```python
from build123d import *

# Parameters (mm, degrees)
SKETCH2_W           = 32.5
SKETCH2_H           = 32.5
SKETCH2_R           = 1
BOSS_EXTRUDE1_DEPTH = 1.5
SKETCH4_W           = 13
SKETCH4_H           = 13
BOSS_EXTRUDE2_DEPTH = 4
SKETCH6_W           = 10
SKETCH6_H           = 4.75
BOSS_EXTRUDE3_DEPTH = 6


with BuildPart() as part:
    # Sketch2 → Boss-Extrude1 (new body)
    with BuildSketch(Plane.XY):
        Rectangle(SKETCH2_W, SKETCH2_H)
        with Locations((13.875, 13.875)):
            Circle(SKETCH2_R, mode=Mode.SUBTRACT)
        with Locations((13.875, -13.875)):
            Circle(SKETCH2_R, mode=Mode.SUBTRACT)
        with Locations((-13.875, -13.875)):
            Circle(SKETCH2_R, mode=Mode.SUBTRACT)
        with Locations((-13.875, 13.875)):
            Circle(SKETCH2_R, mode=Mode.SUBTRACT)
    extrude(amount=BOSS_EXTRUDE1_DEPTH)

    # Sketch4 → Boss-Extrude2 (add)
    with BuildSketch(Plane.XY.offset(1.5)):
        Rectangle(SKETCH4_W, SKETCH4_H)
        with BuildLine():
            Line((8.925, -1.85), (-8.925, -1.85))
            ThreePointArc((-8.925, -1.85), (-10.775, 0), (-8.925, 1.85))
            Line((-8.925, 1.85), (8.925, 1.85))
            ThreePointArc((8.925, 1.85), (10.775, 0), (8.925, -1.85))
        make_face()
    extrude(amount=BOSS_EXTRUDE2_DEPTH)

    # Sketch5 → Revolve1 (revolve)
    with BuildSketch(Plane(origin=(0, 0, 0), x_dir=(1, 0, 0), z_dir=(0, 1, 0)), mode=Mode.PRIVATE) as revolve1_sk:
        with BuildLine():
            Line((0, -5.5), (6.5, -5.5))
            Line((6.5, -5.5), (6.5, -13.4))
            Line((6.5, -13.4), (5.65, -13.4))
            Line((5.65, -13.4), (5.65, -18.4))
            Line((5.65, -18.4), (8.5, -18.4))
            Line((8.5, -18.4), (8.5, -22.9))
            Line((8.5, -22.9), (7.5, -22.9))
            Line((7.5, -22.9), (7.5, -22.190584114))
            ThreePointArc((7.5, -22.190584114), (3.76673834, -22.722251095), (0, -22.9))
            Line((0, -22.9), (0, -5.5))
        make_face()
    revolve(revolve1_sk.sketch.rotate(Axis((0, 0, 0), (0, 0, 1)), 180), axis=Axis((0, 0, 0), (0, 0, 1)))

    # Sketch6 → Boss-Extrude3 (add)
    with BuildSketch(Plane(origin=(0, 0, 0), x_dir=(-1, 0, 0), z_dir=(0, 0, -1))):
        with Locations((0, -13.875)):
            Rectangle(SKETCH6_W, SKETCH6_H)
    extrude(amount=BOSS_EXTRUDE3_DEPTH)


solid = part.part
```
Geometry check sheet. Reference: the model listing, model coordinates, mm. A direction names the side the tool comes from. Coordinates: 2 decimals unless noted, no trailing zeros. Order: outer loops, then holes, each group sorted by start corner. A loop starts at its lowest first (then second) coordinate and runs counter-clockwise, first axis right, second up.
Item 1: Mould release check, pull along Y, two halves, no side actions. Record for faces 5 (the flat face through (0, 0, 0)), 6 (the flat face through (0, -11.5, -3)), 7 (the cylindrical face through (-4.032, -6.324, 22.54)): released by +Y, released by -Y, zero draft, split by the parting line, or undercut.
Item 2: Section check A-A (y = 0). Enter the section's corners in (x, z) (3 decimals).
Item 3: Section check C-C (z = 4.75). Enter the section's corners in (x, y) (3 decimals).
Item 4: Section check D-D (y = 3.5). Enter the section's corners in (x, z), plus the area to 3 significant figures.
Item 5: Tool access check on faces 1 (the flat face through (8, -1.85, 3)), 2 (the flat face through (-8, 1.85, 3)), 3 (the flat face through (2, 6, 18.4)), 4 (the flat face through (0, -6.5, 3)). Record the directions out of +Z, -Z, +X, -X, +Y, -Y that give a thin tool (end or side, any length) a straight path to the whole face; none if there is none.
Item 6: Depth check by flat-ended pin: pin 1 (1 mm diameter, centred on x = -2.5, z = -1, fed in from +Y); pin 2 (2.5 mm diameter, centred on x = -13.875, y = 13.875, fed in from +Z); pin 3 (1.9 mm diameter, centred on x = -8, z = 3.5, fed in from -Y). Enter the tip coordinate at first touch or a pass-through.
Item 7: Scan lines: line 1 along Y through (x, z) = (-14, 0.25); line 2 along Z through (x, y) = (1.5, -8); line 3 along Y through (x, z) = (-13, 1). Record each from-to range of solid material in increasing order.
Check sheet entries:
1. face 5: zero draft
1. face 6: released by +Y
1. face 7: undercut
2. outline: (-16.25, 0) - (16.25, 0) - (16.25, 1.5) - (10.775, 1.5) - (10.775, 5.5) - (6.5, 5.5) - (6.5, 13.4) - (5.65, 13.4) - (5.65, 18.4) - (8.5, 18.4) - (8.5, 22.9) - (7.5, 22.9) - (7.5, 22.191) arc R40 ccw to (-7.5, 22.191) - (-7.5, 22.9) - (-8.5, 22.9) - (-8.5, 18.4) - (-5.65, 18.4) - (-5.65, 13.4) - (-6.5, 13.4) - (-6.5, 5.5) - (-10.775, 5.5) - (-10.775, 1.5) - (-16.25, 1.5) - close
3. outline: (-8.925, -1.85) - (-6.5, -1.85) - (-6.5, -6.5) - (6.5, -6.5) - (6.5, -1.85) - (8.925, -1.85) arc R1.85 ccw to (8.925, 1.85) - (6.5, 1.85) - (6.5, 6.5) - (-6.5, 6.5) - (-6.5, 1.85) - (-8.925, 1.85) arc R1.85 ccw to start
4. outline: (-16.25, 0) - (16.25, 0) - (16.25, 1.5) - (6.5, 1.5) - (6.5, 5.5) - (5.48, 5.5) - (5.48, 13.4) - (4.44, 13.4) - (4.44, 18.4) - (7.75, 18.4) - (7.75, 22.9) - (6.63, 22.9) - (6.63, 22.19) arc R39.85 ccw to (-6.63, 22.19) - (-6.63, 22.9) - (-7.75, 22.9) - (-7.75, 18.4) - (-4.44, 18.4) - (-4.44, 13.4) - (-5.48, 13.4) - (-5.48, 5.5) - (-6.5, 5.5) - (-6.5, 1.5) - (-16.25, 1.5) - close
4. area: 297 mm2
5. face 1: +X, -Y
5. face 2: -X, +Y
5. face 3: none
5. face 4: +X, -X, -Y
6. pin 1: stops at y = -11.5
6. pin 2: stops at z = 1.5
6. pin 3: stops at y = -1.85
7. line 1: y = -16.25 to -14.87, -12.88 to 12.88, 14.87 to 16.25
7. line 2: z = 0 to 1.5, 18.4 to 22.9
7. line 3: y = -16.25 to -14.36, -13.39 to 13.39, 14.36 to 16.25
